```python
from build123d import *

# Parameters (mm, degrees)
F1_DEPTH = 5
F2_W     = 76.953554
F2_H     = 5
F2_W_2   = 74.162988
F3_DEPTH = 14.3
F4_R     = 2.0828
F5_DEPTH = 41.121068
F6_W     = 20.32
F6_H     = 9.22
F7_DEPTH = 41.121068


with BuildPart() as f1:
    # F0 (on Front) → F1 (new body)
    with BuildSketch(Plane.XZ):
        with BuildLine():
            Line((-3.313402, 41.320068), (-0.073779, 0.920068))
            ThreePointArc((-0.073779, 0.920068), (0.244763, 0.265176), (0.923021, 0))
            Line((0.923021, 0), (84.276979, 0))
            ThreePointArc((84.276979, 0), (84.955237, 0.265176), (85.273779, 0.920068))
            Line((85.273779, 0.920068), (88.513402, 41.320068))
            ThreePointArc((88.513402, 41.320068), (88.251425, 42.078258), (87.516601, 42.4))
            Line((87.516601, 42.4), (-2.316601, 42.4))
            ThreePointArc((-2.316601, 42.4), (-3.051425, 42.078258), (-3.313402, 41.320068))
        make_face()
        with BuildLine():
            ThreePointArc((-0.860778, 29.500339), (0.449104, 33.29129), (4.123223, 34.9))
            Line((4.123223, 34.9), (81.076777, 34.9))
            ThreePointArc((81.076777, 34.9), (84.750896, 33.29129), (86.060778, 29.500339))
            Line((86.060778, 29.500339), (84.665495, 12.100339))
            ThreePointArc((84.665495, 12.100339), (83.072784, 8.825881), (79.681494, 7.5))
            Line((79.681494, 7.5), (5.518506, 7.5))
            ThreePointArc((5.518506, 7.5), (2.127216, 8.825881), (0.534505, 12.100339))
            Line((0.534505, 12.100339), (-0.860778, 29.500339))
        make_face(mode=Mode.SUBTRACT)
    extrude(amount=F1_DEPTH)

    # F2 (on face) → F3 (join)
    with BuildSketch(Plane(origin=(0, 0, 0), x_dir=(-1, 0, 0), z_dir=(0, 1, 0))):
        with Locations((-42.6, 38.620068)):
            Rectangle(F2_W, F2_H)
        with Locations((-42.6, 3.620068)):
            Rectangle(F2_W_2, F2_H)
    extrude(amount=F3_DEPTH)

    # F4 (on face) → F5 (cut, through all)
    with BuildSketch(Plane.XY.offset(41.120068)):
        with Locations((24.185, 10.3)):
            Circle(F4_R)
        with Locations((61.015, 10.3)):
            Circle(F4_R)
    extrude(amount=-F5_DEPTH, mode=Mode.SUBTRACT)

    # F6 (on face) → F7 (cut, through all)
    with BuildSketch(Plane.XY.offset(41.120068)):
        Polygon((4.123223, 14.3), (4.123223, 0), (18.093223, 14.3), align=None)
        with Locations((42.604223, 9.69)):
            Rectangle(F6_W, F6_H)
        Polygon((81.076777, 14.3), (67.106777, 14.3), (81.076777, 0), align=None)
    extrude(amount=-F7_DEPTH, mode=Mode.SUBTRACT)


solid = f1.part
```
Geometry check sheet. Reference: the model listing, model coordinates, mm. A direction names the side the tool comes from. Coordinates: 2 decimals unless noted, no trailing zeros. Loops run counter-clockwise (first coordinate to the right, second up) from the corner with the lowest first, then second, coordinate; pieces in that order, holes last.
Item 1: Sectioned sample at B-B, the plane y = -2.25. Record the boundary of the cut face in (x, z), then the cut area to 3 significant figures.
Item 2: Sectioned sample at D-D, the plane y = 10.3. Count the separate pieces of the cut face and the enclosed holes in it, then the cut area to 3 significant figures.
Item 3: Go/stop test with flat-tipped pins: pin 1 Ø5.5 at (x, y) = (24.185, 10.3) entering from -Z; pin 2 Ø4 at (y, z) = (8.5, 38) entering from +X; pin 3 Ø1.5 at (y, z) = (2, 36.5) entering from +X. Record where each tip stops, or that it passes through.
Item 4: Sectioned sample at A-A, the plane x = 56.5. Record the boundary of the cut face in (y, z), then the cut area to 3 significant figures.
Item 5: Thickness scan on line 1 (Z direction, x = 62, y = -3.5); line 2 (X direction, y = 11.5, z = 3.5); line 3 (Z direction, x = 14.5, y = 8). Record the ranges inside material, lowest first.
Item 6: Access from +Z, -Z, +X, -X, +Y, -Y to the whole of each face (thin tool, end or side, straight path). Record for faces 1 (the face through (25, 14.3, 39)), 2 (the face through (22.65, 11.71, 38.66)), 3 (the face through (32.444, 10, 4)), 4 (the face through (42, -2, 34.9)), 5 (the face through (43, 4, 6.12)).
Item 7: Release check for a two-part mould opening along X. For faces 6 (the face through (85, -2, 33)), 7 (the face through (42, -2, 0)), 8 (the face through (73.31, 7.95, 3.66)) record: released by +X, released by -X, zero draft, split by the parting line, or undercut.
Item 8: Sectioned sample at C-C, the plane z = 28. Record the boundary of the cut face in (x, y).
Check result:
1. outline: (-3.31, 41.32) - (-0.07, 0.92) arc R1 ccw to (0.92, 0) - (84.28, 0) arc R1 ccw to (85.27, 0.92) - (88.51, 41.32) arc R1 ccw to (87.52, 42.4) - (-2.32, 42.4) arc R1 ccw to start; hole (-0.86, 29.5) - (0.53, 12.1) arc R5 ccw to (5.52, 7.5) - (79.68, 7.5) arc R5 ccw to (84.67, 12.1) - (86.06, 29.5) arc R5 ccw to (81.08, 34.9) - (4.12, 34.9) arc R5 ccw to start
1. area: 1,430 mm2
2. separate pieces: 8
2. enclosed holes: 0
2. area: 282 mm2
3. pin 1: stops at z = 1.12
3. pin 2: stops at x = 74.73
3. pin 3: stops at x = 79.86
4. outline: (-5, 0) - (0, 0) - (0, 1.12) - (14.3, 1.12) - (14.3, 6.12) - (0, 6.12) - (0, 7.5) - (-5, 7.5) - close; (-5, 34.9) - (0, 34.9) - (0, 36.12) - (14.3, 36.12) - (14.3, 41.12) - (0, 41.12) - (0, 42.4) - (-5, 42.4) - close
4. area: 218 mm2
5. line 1: z = 0 to 7.5, 34.9 to 42.4
5. line 2: x = 15.36 to 22.48, 25.89 to 32.44, 52.76 to 59.31, 62.72 to 69.84
5. line 3: z = 1.12 to 6.12, 36.12 to 41.12
6. face 1: +Z, -Z, +X, -X, +Y
6. face 2: +Z, -Z
6. face 3: +Z, -Z, +Y
6. face 4: +Y, -Y
6. face 5: +X, -X, +Y
7. face 6: undercut
7. face 7: zero draft
7. face 8: released by +X
8. outline: (-2.25, -5) - (-0.74, -5) - (-0.74, 0) - (-2.25, 0) - close; (85.94, -5) - (87.45, -5) - (87.45, 0) - (85.94, 0) - close
